CAD build for the part. Positions are in the model's coordinates, mm. A direction names the side the tool comes from. Round coordinates to 2 decimals unless told otherwise and drop trailing zeros. Order: outer loops, then holes, each group sorted by start corner. A loop starts at its lowest first (then second) coordinate and runs counter-clockwise, first axis right, second up.
```python
from build123d import *

# Parameters (mm, degrees)
F0_R     = 31.75
F1_DEPTH = 50.8
F0_R_2   = 60.325
F2_DEPTH = 12.7
F4_D     = 5.1054
F4_DEPTH = 60.326
F5_R     = 34.925
F6_DEPTH = 3.175
F7_D     = 7.9375


with BuildPart() as f1:
    # F0 (on Top) → F1 (new body)
    with BuildSketch(Plane.XY):
        Circle(F0_R)
        with BuildLine():
            ThreePointArc((4.7625, 20.0869892361), (16.1939012972, 12.80336298), (20.64385, 0))
            ThreePointArc((20.64385, 0), (-12.80336298, -16.1939012972), (-4.7625, 20.0869892361))
            Line((-4.7625, 20.0869892361), (-4.7625, 25.40635))
            Line((-4.7625, 25.40635), (4.7625, 25.40635))
            Line((4.7625, 25.40635), (4.7625, 20.0869892361))
        make_face(mode=Mode.SUBTRACT)
    extrude(amount=F1_DEPTH)

    # F0 (on Top) → F2 (join)
    with BuildSketch(Plane.XY):
        Circle(F0_R_2)
        Circle(F0_R, mode=Mode.SUBTRACT)
        Circle(F0_R)
        with BuildLine():
            ThreePointArc((4.7625, 20.0869892361), (16.1939012972, 12.80336298), (20.64385, 0))
            ThreePointArc((20.64385, 0), (-12.80336298, -16.1939012972), (-4.7625, 20.0869892361))
            Line((-4.7625, 20.0869892361), (-4.7625, 25.40635))
            Line((-4.7625, 25.40635), (4.7625, 25.40635))
            Line((4.7625, 25.40635), (4.7625, 20.0869892361))
        make_face(mode=Mode.SUBTRACT)
    extrude(amount=-F2_DEPTH)

    # F4 (through all, one way)
    with BuildSketch(Plane.XZ):
        with Locations((0, 38.1), (0, 19.05)):
            Circle(F4_D / 2)
    extrude(amount=-F4_DEPTH, mode=Mode.SUBTRACT)

    # F5 (on face) → F6 (cut)
    with BuildSketch(Plane(origin=(0, 0, -12.7), x_dir=(1, 0, 0), z_dir=(0, 0, -1))):
        Circle(F5_R)
        with BuildLine():
            ThreePointArc((-4.7625, -20.0869892361), (0, 20.64385), (4.7625, -20.0869892361))
            Line((4.7625, -20.0869892361), (4.7625, -25.40635))
            Line((4.7625, -25.40635), (-4.7625, -25.40635))
            Line((-4.7625, -25.40635), (-4.7625, -20.0869892361))
        make_face(mode=Mode.SUBTRACT)
    extrude(amount=-F6_DEPTH, mode=Mode.SUBTRACT)

    # F7 (through all)
    with Locations(Plane.XY):
        with Locations((-36.576, -30.734), (36.576, -30.734), (36.576, 30.734), (-36.576, 30.734)):
            Hole(F7_D / 2)


solid = f1.part
```
1. Tool access for faces 1 (the face through (-4.762, 23, 21)), 2 (the face through (-27.715, 21.251, -11.135)), 3 (the face through (-0.553, 28.534, 35.608)), 4 (the face through (-6.883, -30.995, 25.044)): list every direction of +Z, -Z, +X, -X, +Y, -Y with a clear straight run to the whole face (end or side of a thin tool).
2. Cut at C-C, the plane z = 25. Write the cut outline in (x, y).
3. Cut at A-A, the plane x = 0. Write the cut outline in (y, z) (3 decimals), and give its area (3 significant figures).
4. Cut at D-D, the plane x = -28. Write the cut outline in (y, z) (3 decimals).
5. Mould opens along Y. For faces 5 (the face through (26, -26, 0)), 6 (the face through (4.762, 23, 21)), 7 (the face through (-60.267, 2.652, -6.261)) say: released by +Y, released by -Y, zero draft, split by the parting line, or undercut.
6. Cut at B-B, the plane y = 7.5. Write the cut outline in (x, z) (3 decimals), and give its area (3 significant figures).
7. Pin check, flat tips, straight feed: P1, Ø10, axis at x = 15.5, y = 25.5, coming from the -Z side (3 decimals); P2, Ø12, axis at y = 17.5, z = 7.5, coming from the -X side; P3, Ø10, axis at x = 17.5, z = -0.5, coming from the -Y side; P4, Ø10.5, axis at x = -36.576, y = -30.734, coming from the -Z side. Stop position of each tip, or through.
8. Drill centre lines: line 1 (Z direction, x = 0, y = 29.5) (3 decimals); line 2 (Y direction, x = 1, z = 23.5); line 3 (Z direction, x = -3.5, y = -31) (3 decimals). Where is each one in solid material? Low to high.
Outcome:
1. face 1: +Z, -Z
1. face 2: -Z
1. face 3: +Y
1. face 4: +Z
2. outline: circle Ø63.5 at (0, 0); hole (-4.76, 20.09) arc R20.64 ccw (long way) to (4.76, 20.09) - (4.76, 25.41) - (-4.76, 25.41) - close
3. outline: (-60.325, -12.7) - (-34.925, -12.7) - (-34.925, -9.525) - (-20.644, -9.525) - (-20.644, 50.8) - (-31.75, 50.8) - (-31.75, 0) - (-60.325, 0) - close; (25.406, -9.525) - (34.925, -9.525) - (34.925, -12.7) - (60.325, -12.7) - (60.325, 0) - (31.75, 0) - (31.75, 16.497) - (25.406, 16.497) - close; (25.406, 21.603) - (31.75, 21.603) - (31.75, 35.547) - (25.406, 35.547) - close; (25.406, 40.653) - (31.75, 40.653) - (31.75, 50.8) - (25.406, 50.8) - close
3. area: 1,690 mm2
4. outline: (-53.433, -12.7) - (-20.875, -12.7) - (-20.875, -9.525) - (20.875, -9.525) - (20.875, -12.7) - (53.433, -12.7) - (53.433, 0) - (14.969, 0) - (14.969, 50.8) - (-14.969, 50.8) - (-14.969, 0) - (-53.433, 0) - close
5. face 5: zero draft
5. face 6: undercut
5. face 7: split by the parting line
6. outline: (-59.857, -12.7) - (-34.11, -12.7) - (-34.11, -9.525) - (-19.233, -9.525) - (-19.233, 50.8) - (-30.851, 50.8) - (-30.851, 0) - (-59.857, 0) - close; (19.233, -9.525) - (34.11, -9.525) - (34.11, -12.7) - (59.857, -12.7) - (59.857, 0) - (30.851, 0) - (30.851, 50.8) - (19.233, 50.8) - close
6. area: 2,120 mm2
7. P1: stops at z = -9.525
7. P2: stops at x = -29.59
7. P3: stops at y = -59.02
7. P4: stops at z = -12.7
8. line 1: z = -9.525 to 16.497, 21.603 to 35.547, 40.653 to 50.8
8. line 2: y = -31.73 to -20.62, 25.41 to 31.73
8. line 3: z = -9.525 to 50.8
